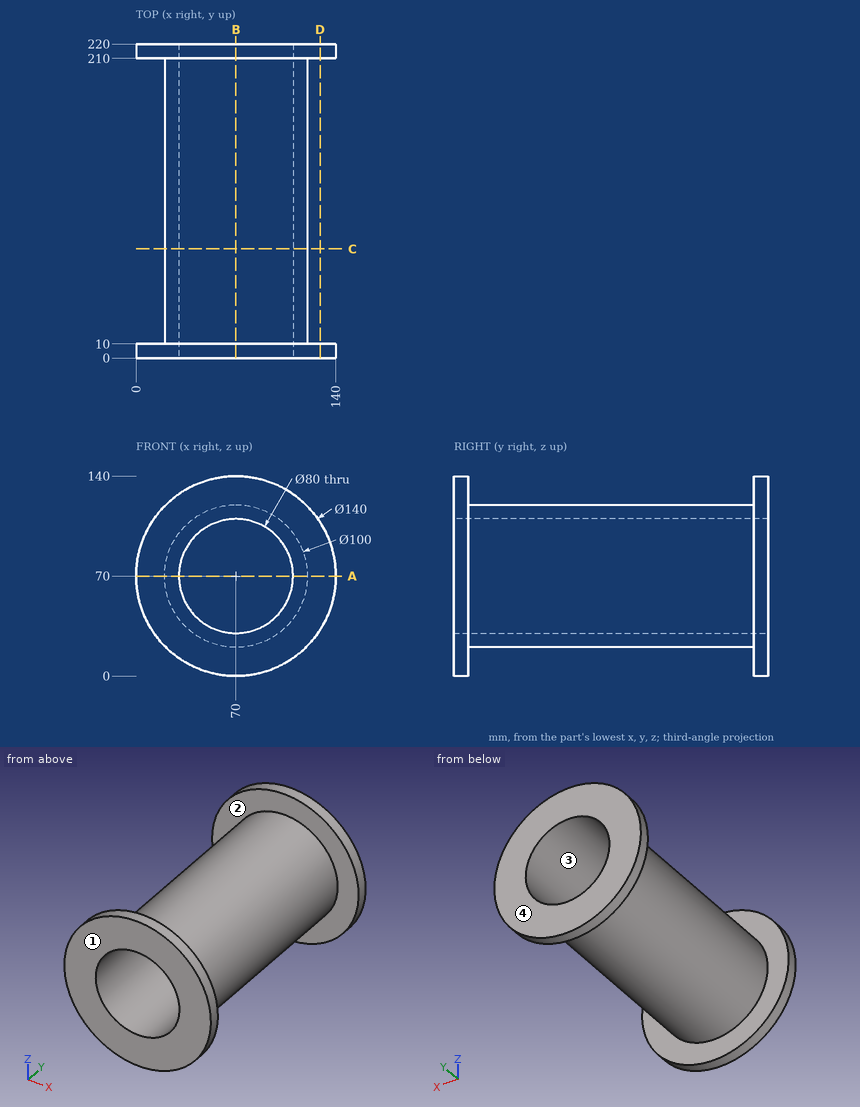
Could you check a few things on this drawing? It's one solid part, dimensions in mm from its lowest x, y, z. Round coordinates to 2 decimals unless told otherwise and drop trailing zeros. Write each loop counter-clockwise with the first axis right and the second up, starting at its lowest first coordinate (ties: lowest second). Pieces come first, ordered by that corner, then holes. Notation, with made-up numbers: (-31, 47) -> (26, 47) arc R19 cw to (26, 59) -> close; hole circle Ø5 at (-35, -28). An arc over 180 degrees is marked (long way). One line per question, with ' | ' between items. Start each with the question number.
1) I need wall thicknesses on line 1 (X direction, y = 160, z = 70); line 2 (Y direction, x = 134, z = 63.5); line 3 (X direction, y = 141, z = 92). Which ranges of each line are inside material? Lowest first, please. Write a range as [from, to].
2) If we mould it in two halves opening along Y, with no side actions, what happens to the marked faces 1, 2, 3 and 4? For each: released by +Y, released by -Y, zero draft, split by the parting line, or undercut.
3) I'm going to push flat-ended pins straight in: P1, Ø1, axis at x = 61, y = 24.5, coming from the +Z side; P2, Ø3, axis at x = 85.5, y = 161.5, coming from the +Z side; P3, Ø3, axis at x = 36.5, y = 75.5, coming from the +Z side. Where does each tip first touch, or does it pass through?
4) Suppose I cut it at B-B on x = 70. Write out the boundary of the cut face in (y, z), then the cut area to 3 significant figures.
5) Suppose I cut it at C-C on y = 76.5. Write out the boundary of the cut face in (x, z).
6) Suppose I cut it at A-A on z = 70. Write out the boundary of the cut face in (x, y), then the cut area to 3 significant figures.
7) Suppose I cut it at D-D on x = 129. Write out the boundary of the cut face in (y, z), then the cut area to 3 significant figures.
Return value:
1) line 1: x = [20, 30], [110, 120] | line 2: y = [0, 10], [210, 220] | line 3: x = [25.1, 36.59], [103.41, 114.9]
2) face 1: released by -Y | face 2: undercut | face 3: zero draft | face 4: released by +Y
3) P1: stops at z = 119.27 | P2: stops at z = 118 | P3: stops at z = 108.42
4) outline: (0, 0) -> (10, 0) -> (10, 20) -> (210, 20) -> (210, 0) -> (220, 0) -> (220, 30) -> (0, 30) -> close; (0, 110) -> (220, 110) -> (220, 140) -> (210, 140) -> (210, 120) -> (10, 120) -> (10, 140) -> (0, 140) -> close | area: 5,200 mm2
5) outline: circle Ø100 at (70, 70); hole circle Ø80 at (70, 70)
6) outline: (0, 0) -> (30, 0) -> (30, 220) -> (0, 220) -> (0, 210) -> (20, 210) -> (20, 10) -> (0, 10) -> close; (110, 0) -> (140, 0) -> (140, 10) -> (120, 10) -> (120, 210) -> (140, 210) -> (140, 220) -> (110, 220) -> close | area: 5,200 mm2
7) outline: (0, 32.33) -> (10, 32.33) -> (10, 107.67) -> (0, 107.67) -> close; (210, 32.33) -> (220, 32.33) -> (220, 107.67) -> (210, 107.67) -> close | area: 1,510 mm2
